```python
from build123d import *

# Parameters (mm, degrees)
BOSS_EXTRUDE1_DEPTH = 19.05
SKETCH2_R           = 3.3782
CUT_EXTRUDE1_DEPTH  = 42.311259545
FILLET1_R           = 3.175


with BuildPart() as part:
    # Sketch1 → Boss-Extrude1 (new body)
    with BuildSketch(Plane.XY):
        with BuildLine():
            Line((14.2875, 0), (33.3375, 0))
            Line((33.3375, 0), (33.3375, 6.35))
            Line((33.3375, 6.35), (20.6375, 6.35))
            ThreePointArc((20.6375, 6.35), (0, 21.592334433), (-20.6375, 6.35))
            Line((-20.6375, 6.35), (-33.3375, 6.35))
            Line((-33.3375, 6.35), (-33.3375, 0))
            Line((-33.3375, 0), (-14.2875, 0))
            ThreePointArc((-14.2875, 0), (0, 14.2875), (14.2875, 0))
        make_face()
    extrude(amount=BOSS_EXTRUDE1_DEPTH)

    # Sketch2 → Cut-Extrude1 (cut, through all)
    with BuildSketch(Plane(origin=(0, 6.35, 0), x_dir=(1, 0, 0), z_dir=(0, 1, 0))):
        with Locations(Location((26.9875, -9.525, 0), (0, 0, 180))):
            Circle(SKETCH2_R)
        with Locations(Location((-26.9875, -9.525, 0), (0, 0, 180))):
            Circle(SKETCH2_R)
    extrude(amount=-CUT_EXTRUDE1_DEPTH, mode=Mode.SUBTRACT)

    # Fillet1
    fillet1_edges = [part.edges().sort_by_distance(p)[0] for p in [
        (-14.2875, 0, 9.525),
        (14.2875, 0, 9.525),
    ]]
    fillet(fillet1_edges, radius=FILLET1_R)


solid = part.part
```
Source: CAD feature listing. Evaluate the final solid. Frame: model axes, mm. A direction names the side the tool comes from. Round coordinates to 2 decimals unless told otherwise and drop trailing zeros. Write each loop counter-clockwise with the first axis right and the second up, starting at its lowest first coordinate (ties: lowest second). Pieces come first, ordered by that corner, then holes. Notation, with made-up numbers: M -3,-15 L 37,-15 A26 ccw 37,1 Z; hole C 32,32.5 d7. An arc over 180 degrees is marked long. Answer as a JSON object with one key per item and string values. Group by question number.
(1) Reachability of faces 4 (the cylindrical face through (-15.12, 0.75, 9.66)), 5 (the flat face through (30, 6.35, 7)), 6 (the flat face through (-24, 6.35, 7)) from +Z, -Z, +X, -X, +Y, -Y: full face, straight path, thin tool, end or side. Return the list, or none.
(2) Ray query, line 1 (Y direction, x = 28, z = 4.25); line 2 (X direction, y = 2, z = 1.5); line 3 (X direction, y = 8.25, z = 5). Return the intervals inside material, ascending. Write a range as [from, to].
(3) Section query A-A on y = 13.25. Output: boundary loops of the cut face in (x, z), then the cut area to 3 significant figures.
(4) Mould query, pull axis Z, two halves, no side actions, for faces 1 (the cylindrical face through (-0.278, 14.285, 9.392)), 2 (the cylindrical face through (-30.21, 3.22, 10.54)), 3 (the flat face through (0, 16, 19.05)). Classes: +Z half, -Z half, draft (parallel to the pull), parting line (faces both ways), or undercut.
(5) First-contact query: pin 1 (2 mm diameter, centred on x = 9, z = 6, fed in from +Y); pin 2 (1 mm diameter, centred on y = 11.5, z = 16, fed in from -X); pin 3 (4 mm diameter, centred on y = 15, z = 11.5, fed in from -X). Flat tips, straight axial feed; report the tip coordinate or a pass-through.
(6) Section query C-C on z = 8.25. State how many separate pieces and enclosed holes the cut face has, then the cut area to 3 significant figures.
(7) Section query B-B on x = -28. Output: boundary loops of the cut face in (y, z), then the cut area to 3 significant figures.
Computed values:
{
 "1": {"face 4": "+Z, -Z, -Y", "face 5": "+Z, -Z, +X, +Y", "face 6": "+Z, -Z, -X, +Y"},
 "2": {"line 1": "[0, 6.35]", "line 2": "[-33.34, -14.22], [14.22, 33.34]", "line 3": "[-19.95, -11.66], [11.66, 19.95]"},
 "3": {"outline": "M -17.05,0 L -5.35,0 L -5.35,19.05 L -17.05,19.05 Z; M 5.35,0 L 17.05,0 L 17.05,19.05 L 5.35,19.05 Z", "area": "446 mm^2"},
 "4": {"face 1": "draft", "face 2": "undercut", "face 3": "+Z half"},
 "5": {"pin 1": "y = 20.06", "pin 2": "x = -18.58", "pin 3": "x = -17.24"},
 "6": {"separate pieces": "3", "enclosed holes": "0", "area": "482 mm^2"},
 "7": {"outline": "M 0,0 L 6.35,0 L 6.35,6.3 L 0,6.3 Z; M 0,12.75 L 6.35,12.75 L 6.35,19.05 L 0,19.05 Z", "area": "80.0 mm^2"}
}
